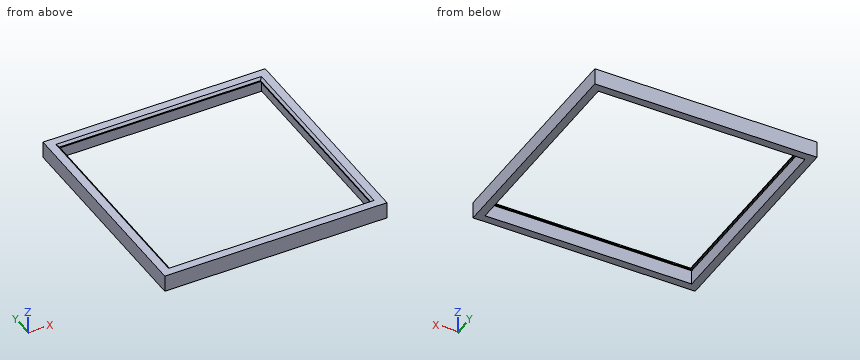
Autodesk Inventor part; units mm, degrees
ref_plane "YZ Plane" through (0, 0, 0) normal (1, 0, 0) x (0, 1, 0)
ref_plane "XZ Plane" through (0, 0, 0) normal (0, 1, 0) x (-1, 0, 0)
ref_plane "XY Plane" through (0, 0, 0) normal (0, 0, 1) x (1, 0, 0)
sketch "Szkic1" plane through (0, 0, 0) normal (0, 0, 1) x (1, 0, 0)
  line L0 (500, -500) -> (-500, -500)
  line L1 (-500, -500) -> (-500, 500)
  line L2 (-500, 500) -> (500, 500)
  line L3 (500, 500) -> (500, -500)
  line L4 (500, -500) -> (-500, 500) construction
  line L5 (-500, -500) -> (500, 500) construction
  line L6 (465, -465) -> (-465, -465)
  line L7 (-465, -465) -> (-465, 465)
  line L8 (-465, 465) -> (465, 465)
  line L9 (465, 465) -> (465, -465)
  line L10 (465, -465) -> (-465, 465) construction
  line L11 (-465, -465) -> (465, 465) construction
  point P0 (0, 0)
  dimension "d0" = 1000
  dimension "d1" = 1000
  dimension "d2" = 930
  dimension "d3" = 930
extrude "Wyciągnięcie proste1" add sketch "Szkic1" along normal mid plane 75
sketch "Szkic2" plane through (0, 0, 37.5) normal (0, 0, 1) x (1, 0, 0)
  line L0 (465, -465) -> (465, 465)
  line L1 (-465, 465) -> (465, 465)
  line L2 (465, 465) -> (465, -465)
  line L3 (465, -465) -> (-465, -465)
  line L4 (-465, -465) -> (-465, 465)
  line L5 (-465, 465) -> (465, -465) construction
  line L6 (465, 465) -> (-465, -465) construction
  line L7 (-452.5, 452.5) -> (452.5, 452.5)
  line L8 (452.5, 452.5) -> (452.5, -452.5)
  line L9 (452.5, -452.5) -> (-452.5, -452.5)
  line L10 (-452.5, -452.5) -> (-452.5, 452.5)
  line L11 (-452.5, 452.5) -> (452.5, -452.5) construction
  line L12 (452.5, 452.5) -> (-452.5, -452.5) construction
  point P0 (0, 0)
  dimension "d6" = 905
  dimension "d7" = 905
extrude "Wyciągnięcie proste2" add sketch "Szkic2" against normal blind 10
chamfer "Faza1" distance 10 angle 45 4 edges at (452.5, 0, 37.5) (0, 452.5, 37.5) (-452.5, 0, 37.5) (0, -452.5, 37.5)
ref_plane "Płaszczyzna konstrukcyjna1" through (-452.5, 452.5, 27.5) normal (0, 0, 1) x (0, -1, 0)
sketch "Szkic3" plane through (0, 0, 27.5) normal (0, 0, -1) x (-1, 0, 0)
  line L0 (452.5, 452.5) -> (452.5, -452.5)
  line L1 (-452.5, -452.5) -> (452.5, -452.5)
  line L2 (452.5, -452.5) -> (452.5, 452.5)
  line L3 (452.5, 452.5) -> (-452.5, 452.5)
  line L4 (-452.5, 452.5) -> (-452.5, -452.5)
  line L5 (-452.5, -452.5) -> (452.5, 452.5) construction
  line L6 (452.5, -452.5) -> (-452.5, 452.5) construction
  line L7 (-457.5, -457.5) -> (457.5, -457.5)
  line L8 (457.5, -457.5) -> (457.5, 457.5)
  line L9 (457.5, 457.5) -> (-457.5, 457.5)
  line L10 (-457.5, 457.5) -> (-457.5, -457.5)
  line L11 (-457.5, -457.5) -> (457.5, 457.5) construction
  line L12 (457.5, -457.5) -> (-457.5, 457.5) construction
  point P0 (0, 0)
  dimension "d13" = 915
extrude "Wyciągnięcie proste3" add sketch "Szkic3" along normal blind 5
properties part number "rama" material "Tworzywo sztuczne PC/ABS"
Geometry check sheet. Reference: the model listing, model coordinates, mm. Round coordinates to 2 decimals unless told otherwise and drop trailing zeros. Loops run counter-clockwise (first coordinate to the right, second up) from the corner with the lowest first, then second, coordinate; pieces in that order, holes last.
Item 1: Thickness scan on line 1 (Y direction, x = 322, z = 25); line 2 (Y direction, x = -394, z = 15). Record the ranges inside material, lowest first.
Item 2: Cross-section at C-C on z = -10. Record the boundary of the cut face in (x, y), then the cut area to 3 significant figures.
Item 3: Cross-section at A-A on y = -370. Record the boundary of the cut face in (x, z), then the cut area to 3 significant figures.
Answer sheet:
1. line 1: y = -500 to -465, -457.5 to -452.5, 452.5 to 457.5, 465 to 500
1. line 2: y = -500 to -465, 465 to 500
2. outline: (-500, -500) - (500, -500) - (500, 500) - (-500, 500) - close; hole (-465, -465) - (465, -465) - (465, 465) - (-465, 465) - close
2. area: 135,000 mm2
3. outline: (-500, -37.5) - (-465, -37.5) - (-465, 27.5) - (-457.5, 27.5) - (-457.5, 22.5) - (-452.5, 22.5) - (-452.5, 27.5) - (-462.5, 37.5) - (-500, 37.5) - close; (452.5, 22.5) - (457.5, 22.5) - (457.5, 27.5) - (465, 27.5) - (465, -37.5) - (500, -37.5) - (500, 37.5) - (462.5, 37.5) - (452.5, 27.5) - close
3. area: 5,450 mm2
